```python
from build123d import *

# Parameters (mm, degrees)
F0_W      = 16
F0_H      = 3
F0_H_2    = 10
F0_W_2    = 9.5
F0_R      = 1.5
F0_H_3    = 5
F1_DEPTH  = 3
F3_DEPTH  = 9
F5_DEPTH  = 18.001
F7_DEPTH  = 1
F9_DEPTH  = 1
F11_DEPTH = 1
F13_DEPTH = 1
F14_W     = 3
F14_H     = 1
F14_H_2   = 9
F15_DEPTH = 10


with BuildPart() as f1:
    # F0 (on Top) → F1 (new body)
    with BuildSketch(Plane.XY):
        with Locations((-2.323942259, 4.8155895834)):
            Rectangle(F0_W, F0_H)
        with Locations((-2.323942259, -1.6844104166)):
            Rectangle(F0_W, F0_H_2)
        with Locations((-15.073942259, -1.6844104166)):
            Rectangle(F0_W_2, F0_H_2)
        with Locations((-14.823942259, -1.6844104166)):
            Circle(F0_R, mode=Mode.SUBTRACT)
        with Locations((-2.323942259, -9.1844104166)):
            Rectangle(F0_W, F0_H_3)
        with Locations((10.426057741, -1.6844104166)):
            Rectangle(F0_W_2, F0_H_2)
        with Locations((10.176057741, -1.6844104166)):
            Circle(F0_R, mode=Mode.SUBTRACT)
    extrude(amount=F1_DEPTH)

    # F2 (on face) → F3 (join)
    with BuildSketch(Plane.XY.offset(3)):
        Polygon((-10.323942259, -6.6844104166), (-10.323942259, -11.6844104166), (5.676057741, -11.6844104166), (5.676057741, -6.6844104166), (5.676057741, 3.3155895834), (5.676057741, 6.3155895834), (-10.323942259, 6.3155895834), (-10.323942259, 3.3155895834), align=None)
    extrude(amount=F3_DEPTH)

    # F4 (on face) → F5 (cut, through all)
    with BuildSketch(Plane.XZ.offset(11.6844104166)):
        with BuildLine():
            ThreePointArc((-5.323942259, 10), (-7.4452626025, 9.1213203436), (-8.323942259, 7))
            ThreePointArc((-8.323942259, 7), (-5.323942259, 4), (-2.323942259, 7))
            ThreePointArc((-2.323942259, 7), (-3.2026219154, 9.1213203436), (-5.323942259, 10))
        make_face()
        with BuildLine():
            Line((0.6760577337, 10), (-5.323942259, 10))
            ThreePointArc((-5.323942259, 10), (-3.2026219154, 9.1213203436), (-2.323942259, 7))
            ThreePointArc((-2.323942259, 7), (-1.4452626051, 9.121320341), (0.6760577337, 10))
        make_face()
        with BuildLine():
            ThreePointArc((-2.323942259, 7), (0.676057741, 4), (3.676057741, 7))
            ThreePointArc((3.676057741, 7), (2.797378082, 9.1213203461), (0.6760577337, 10))
            ThreePointArc((0.6760577337, 10), (-1.4452626051, 9.121320341), (-2.323942259, 7))
        make_face()
        with BuildLine():
            Line((-8.323942259, 7), (-8.323942259, 0))
            Line((-8.323942259, 0), (3.676057741, 0))
            Line((3.676057741, 0), (3.676057741, 7))
            ThreePointArc((3.676057741, 7), (0.676057741, 4), (-2.323942259, 7))
            ThreePointArc((-2.323942259, 7), (-5.323942259, 4), (-8.323942259, 7))
        make_face()
    extrude(amount=-F5_DEPTH, mode=Mode.SUBTRACT)

    # F6 (on face) → F7 (join)
    with BuildSketch(Plane.XZ.offset(6.6844104166)):
        Polygon((-10.323942259, 12), (-19.823942259, 3), (-10.323942259, 3), align=None)
    extrude(amount=-F7_DEPTH)

    # F8 (on face) → F9 (join)
    with BuildSketch(Plane(origin=(0, 3.3155895834, 0), x_dir=(-1, 0, 0), z_dir=(0, 1, 0))):
        Polygon((10.323942259, 3), (19.823942259, 3), (10.323942259, 12), align=None)
    extrude(amount=-F9_DEPTH)

    # F10 (on face) → F11 (join)
    with BuildSketch(Plane(origin=(0, 3.3155895834, 0), x_dir=(-1, 0, 0), z_dir=(0, 1, 0))):
        Polygon((-5.676057741, 12), (-15.176057741, 3), (-5.676057741, 3), align=None)
    extrude(amount=-F11_DEPTH)

    # F12 (on face) → F13 (join)
    with BuildSketch(Plane.XZ.offset(6.6844104166)):
        Polygon((5.676057741, 3), (15.176057741, 3), (5.676057741, 12), align=None)
    extrude(amount=-F13_DEPTH)

    # F14 (on face) → F15 (cut)
    with BuildSketch(Plane(origin=(0, 0, 0), x_dir=(1, 0, 0), z_dir=(0, 0, -1))):
        with Locations((-6.823942259, -0.8155895834)):
            Rectangle(F14_W, F14_H)
        with Locations((-6.823942259, -5.8155895834)):
            Rectangle(F14_W, F14_H)
        with Locations((2.176057741, -1.8155895834)):
            Rectangle(F14_W, F14_H_2)
        with Locations((-6.823942259, 2.1844104166)):
            Rectangle(F14_W, F14_H)
    extrude(amount=-F15_DEPTH, mode=Mode.SUBTRACT)


solid = f1.part
```
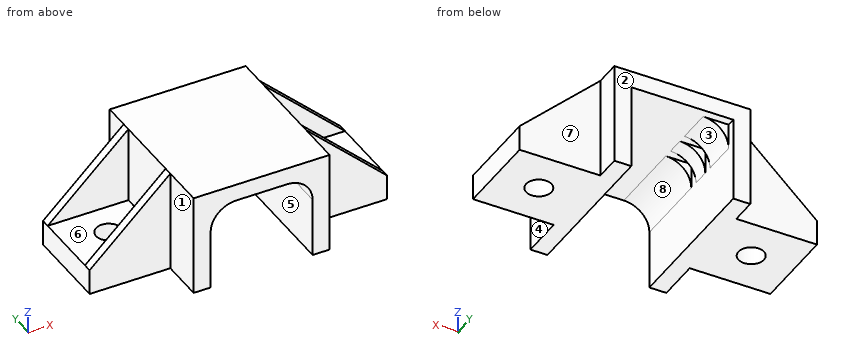
Geometry: final body of the model. Coordinates: model frame, mm. Face numbers are marked on the shaded views. A direction names the side the tool comes from. Coordinates: 2 decimals unless noted, no trailing zeros. Loops run counter-clockwise (first coordinate to the right, second up) from the corner with the lowest first, then second, coordinate; pieces in that order, holes last. Notation, with made-up numbers: (12, -24) -> (18, -24) arc R21 ccw to (18, -12) -> close; hole circle Ø8 at (76.25, 11). An arc over 180 degrees is marked (long way). Use a Markdown table: item, result. Add a question column.
(1) Mould query, pull axis X, two halves, no side actions, for the marked faces 1, 2 and 3. Classes: pulls with the +X half, pulls with the -X half, needs draft (parallel to the pull), parting line crosses it, or undercut.
(2) Access query for the marked faces 4, 5, 6, 7 and 8. Directions: +Z, -Z, +X, -X, +Y, -Y. A direction counts if a zero-diameter tool reaches every point of the face in a straight line with its end or side. Return the directions, or none.
(3) Line query: line 1 along Y through (x, z) = (9, 6); line 2 along X through (y, z) = (-4, 6.75); line 3 along Z through (x, y) = (9, -4.75). Output: solid intervals per line, ascending.
(4) Section query D-D, the plane x = 12.5. Return loops of the section in (y, z).
(5) Pin query (flat end, axial travel): pin 1 Ø3 at (x, z) = (1, 3) entering from -Y; pin 2 Ø1.5 at (y, z) = (-6.5, 7) entering from +X; pin 3 Ø5 at (x, z) = (10.5, 6.5) entering from -Y; pin 4 Ø3 at (x, z) = (3.5, 7.5) entering from +Y. Return the tip coordinate at first contact, or that it passes through.
(6) Section query B-B, the plane z = 3.75. Return loops of the section in (x, y).
(7) Section query A-A, the plane y = -8.25. Return loops of the section in (x, z), plus the area to 3 significant figures.
(8) Section query C-C, the plane x = -15. Return loops of the section in (y, z), plus the area to 3 significant figures.
Answer:
| question | item | result |
|---|---|---|
| 1 | face 1 | pulls with the -X half |
| 1 | face 2 | needs draft |
| 1 | face 3 | undercut |
| 2 | face 4 | +Z, -Z, +X, -Y |
| 2 | face 5 | -Z, +Y |
| 2 | face 6 | +Z, -X |
| 2 | face 7 | +Z, -Z, +X, +Y |
| 2 | face 8 | -Z, +Y, -Y |
| 3 | line 1 | y = -6.68 to -5.68, 2.32 to 3.32 |
| 3 | line 2 | x = -10.32 to -8.32, 3.68 to 5.68 |
| 3 | line 3 | z = 0 to 3 |
| 4 | outline | (-6.68, 0) -> (3.32, 0) -> (3.32, 5.54) -> (2.32, 5.54) -> (2.32, 3) -> (-5.68, 3) -> (-5.68, 5.54) -> (-6.68, 5.54) -> close |
| 5 | pin 1 | passes through |
| 5 | pin 2 | stops at x = 11.75 |
| 5 | pin 3 | stops at y = -6.68 |
| 5 | pin 4 | stops at y = 6.32 |
| 6 | outline | (-19.03, -6.68) -> (-10.32, -6.68) -> (-10.32, -11.68) -> (-8.32, -11.68) -> (-8.32, 6.32) -> (-10.32, 6.32) -> (-10.32, 3.32) -> (-19.03, 3.32) -> (-19.03, 2.32) -> (-10.32, 2.32) -> (-10.32, -5.68) -> (-19.03, -5.68) -> close; (3.68, -11.68) -> (5.68, -11.68) -> (5.68, -6.68) -> (14.38, -6.68) -> (14.38, -5.68) -> (5.68, -5.68) -> (5.68, 2.32) -> (14.38, 2.32) -> (14.38, 3.32) -> (5.68, 3.32) -> (5.68, 6.32) -> (3.68, 6.32) -> close |
| 7 | outline | (-10.32, 0) -> (-8.32, 0) -> (-8.32, 7) arc R3 cw to (-5.32, 10) -> (0.68, 10) arc R3 cw to (3.68, 7) -> (3.68, 0) -> (5.68, 0) -> (5.68, 12) -> (-10.32, 12) -> close |
| 7 | area | 75.9 mm^2 |
| 8 | outline | (-6.68, 0) -> (-3.17, 0) -> (-3.17, 3) -> (-5.68, 3) -> (-5.68, 7.57) -> (-6.68, 7.57) -> close; (-0.19, 0) -> (3.32, 0) -> (3.32, 7.57) -> (2.32, 7.57) -> (2.32, 3) -> (-0.19, 3) -> close |
| 8 | area | 30.2 mm^2 |
